Can you work these out from the model? Positions are in its coordinate system, mm. Face numbers are marked on the shaded views. Give positions to 0.01 mm unless a question says otherwise; leave off trailing zeros. Loops run counter-clockwise (first coordinate to the right, second up) from the corner with the lowest first, then second, coordinate; pieces in that order, holes last. Notation, with made-up numbers: (7.5, 74) -> (54.5, 74) arc R6 ccw to (54.5, 85) -> close; hole circle Ø9 at (42.25, 14). An arc over 180 degrees is marked (long way). Use CSV: the item, a comma, the result in double quotes.
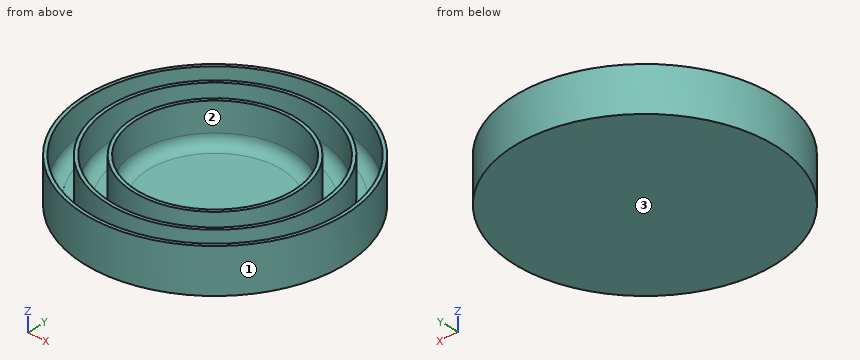
from build123d import *

# Parameters (mm, degrees)
F0_R     = 58.4474221673
F0_R_2   = 56.9474221673
F0_R_3   = 48
F0_R_4   = 46.5
F0_R_5   = 36.5
F0_R_6   = 35
F1_DEPTH = 2
F2_DEPTH = 20
F3_R     = 5


with BuildPart() as f1:
    # F0 (on Top) → F1 (new body)
    with BuildSketch(Plane.XY):
        Circle(F0_R)
        Circle(F0_R_2, mode=Mode.SUBTRACT)
        Circle(F0_R_2)
        Circle(F0_R_3, mode=Mode.SUBTRACT)
        Circle(F0_R_3)
        Circle(F0_R_4, mode=Mode.SUBTRACT)
        Circle(F0_R_4)
        Circle(F0_R_5, mode=Mode.SUBTRACT)
        Circle(F0_R_5)
        Circle(F0_R_6, mode=Mode.SUBTRACT)
        Circle(F0_R_6)
    extrude(amount=F1_DEPTH)

    # F0 (on Top) → F2 (join)
    with BuildSketch(Plane.XY):
        Circle(F0_R)
        Circle(F0_R_2, mode=Mode.SUBTRACT)
        Circle(F0_R_3)
        Circle(F0_R_4, mode=Mode.SUBTRACT)
        Circle(F0_R_5)
        Circle(F0_R_6, mode=Mode.SUBTRACT)
    extrude(amount=F2_DEPTH)

    # F3
    f3_edges = [f1.edges().sort_by_distance(p)[0] for p in [
        (-35, 0, 2),
        (-46.5, 0, 2),
        (-56.947422, 0, 2),
    ]]
    fillet(f3_edges, radius=F3_R)


solid = f1.part
(1) If we section it at D-D, the plane z = 3.75: Write out the boundary of the cut face in (x, y), then the cut area to 3 significant figures.
Answer sheet:
outline,"circle Ø116.89 at (0, 0); circle Ø96 at (0, 0); circle Ø73 at (0, 0); hole circle Ø111.49 at (0, 0); hole circle Ø90.6 at (0, 0); hole circle Ø67.6 at (0, 0)"
area,"2,360 mm2"
(2) If I drill on L1, parallel to Y at x = 0, z = 12.5; L2, parallel to Y at x = -28, z = 15; L3, parallel to X at y = 24, z = 17.25, over which ranges is the centre line in solid material (lowest first)? Write a range as from..to.
Answer sheet:
L1,"y = -58.45..-56.95, -48..-46.5, -36.5..-35, 35..36.5, 46.5..48, 56.95..58.45"
L2,"y = -51.3..-49.59, -38.99..-37.12, -23.41..-21, 21..23.41, 37.12..38.99, 49.59..51.3"
L3,"x = -53.29..-51.64, -41.57..-39.83, -27.5..-25.48, 25.48..27.5, 39.83..41.57, 51.64..53.29"
(3) Will these pins go through, and if not, where does the flat tip stop? pin 1 Ø1.5 at (y, z) = (32, 11) entering from +X; pin 2 Ø1.5 at (y, z) = (-45, 14) entering from -X; pin 3 Ø10 at (y, z) = (32, 16.5) entering from -X.
Answer sheet:
pin 1,"stops at x = 49.39"
pin 2,"stops at x = -38.18"
pin 3,"stops at x = -51.84"
(4) We'd pull the mould along X, two halves only. Please class the marked faces 1, 2 and 3: released by +X, released by -X, zero draft, split by the parting line, or undercut.
Answer sheet:
face 1,"split by the parting line"
face 2,"undercut"
face 3,"zero draft"
(5) If we section it at A-A, the plane z = 13.5: Write out the boundary of the cut face in (x, y), then the cut area to 3 significant figures.
Answer sheet:
outline,"circle Ø116.89 at (0, 0); circle Ø96 at (0, 0); circle Ø73 at (0, 0); hole circle Ø113.89 at (0, 0); hole circle Ø93 at (0, 0); hole circle Ø70 at (0, 0)"
area,"1,330 mm2"
